```python
from build123d import *


with BuildPart() as part:
    # Эскиз1 → Повернуть1 (revolve)
    with BuildSketch(Plane.XZ, mode=Mode.PRIVATE) as revolve_1_sk:
        Polygon((5.053, 0.947), (6, 0), (12.5, 0), (13, 0.5), (13, 59.5), (12.5, 60), (11, 60), (10.5, 59.5), (10.5, 13), (5.053, 12.053), align=None)
    revolve(revolve_1_sk.sketch.rotate(Axis((0, 0, 60.005), (0, 0, -1)), 180), axis=Axis((0, 0, 60.005), (0, 0, -1)))


solid = part.part
```
CAD build for the part. Positions are in the model's coordinates, mm. A direction names the side the tool comes from. Give positions to 0.01 mm unless a question says otherwise; leave off trailing zeros. Write each loop counter-clockwise with the first axis right and the second up, starting at its lowest first coordinate (ties: lowest second). Pieces come first, ordered by that corner, then holes. Notation, with made-up numbers: M 44,18 L 103,18 A5 ccw 103,27 Z; hole C -18.75,-26 d1. An arc over 180 degrees is marked long. Return JSON: item names as keys, results as strings. Group by question number.
(1) Band-saw the part on A-A (y = 0). Give the cut face in (x, z), and give its area (3 significant figures).
(2) Drill centre lines: L1, parallel to Y at x = 0, z = 28; L2, parallel to Y at x = 0, z = 4; L3, parallel to X at y = -3.25, z = 6. Where is each one in solid material? Low to high. Write a range as [from, to].
(3) Mould opens along Y. For faces 3 (the face through (-5, -10, 60)), 4 (the face through (1.15, -5.19, 12.1)), 5 (the face through (10.316, -7.91, 30.413)) say: pulls with the +Y half, pulls with the -Y half, needs draft (parallel to the pull), parting line crosses it, or undercut.
(4) Flat gauge pins, fed straight in: pin 1 Ø12.5 at (x, y) = (0, 0) entering from +Z; pin 2 Ø2 at (y, z) = (-10, 25) entering from -X; pin 3 Ø6 at (x, z) = (-4.5, 37) entering from +Y; pin 4 Ø8 at (x, y) = (0, 0) entering from +Z. Where does each tip first touch, or does it go through?
(5) 3-axis set-ups, long thin cutter, end or side, ignore diameter. For faces 1 (the face through (-10, 3.2, 35.9)), 2 (the face through (0.66, 5.01, 6.42)): which of +Z, -Z, +X, -X, +Y, -Y reach the whole face in a straight line?
(6) Band-saw the part on C-C (z = 39). Give the cut face in (x, y).
Entries:
{
 "1": {"outline": "M -13,0.5 L -12.5,0 L -6,0 L -5.05,0.95 L -5.05,12.05 L -10.5,13 L -10.5,59.5 L -11,60 L -12.5,60 L -13,59.5 Z; M 5.05,0.95 L 6,0 L 12.5,0 L 13,0.5 L 13,59.5 L 12.5,60 L 11,60 L 10.5,59.5 L 10.5,13 L 5.05,12.05 Z", "area": "435 mm^2"},
 "2": {"L1": "y = [-13, -10.5], [10.5, 13]", "L2": "y = [-13, -5.05], [5.05, 13]", "L3": "x = [-12.59, -3.87], [3.87, 12.59]"},
 "3": {"face 3": "needs draft", "face 4": "undercut", "face 5": "parting line crosses it"},
 "4": {"pin 1": "stops at z = 12.26", "pin 2": "stops at x = -9.38", "pin 3": "stops at y = 12.91", "pin 4": "passes through"},
 "5": {"face 1": "+Z", "face 2": "+Z, -Z"},
 "6": {"outline": "C 0,0 d26; hole C 0,0 d21"}
}
